Build history of the part. All positions in model axes, mm. A direction names the side the tool comes from. Round coordinates to 2 decimals unless told otherwise and drop trailing zeros. Write each loop counter-clockwise with the first axis right and the second up, starting at its lowest first coordinate (ties: lowest second). Pieces come first, ordered by that corner, then holes. Notation, with made-up numbers: M 49,60.25 L 81,60.25 A19 ccw 81,70.25 Z; hole C -30,70.25 d3. An arc over 180 degrees is marked long. Use a Markdown table: item, result.
from build123d import *

# Parameters (mm, degrees)
F0_W      = 1.5
F0_H      = 2
F0_H_2    = 12
F0_W_2    = 25
F0_H_3    = 16.5
F1_DEPTH  = 2
F2_DEPTH  = 12
F3_DEPTH  = 4
F4_DEPTH  = 7.97
F5_DEPTH  = 6
F6_SIZE2  = 5
F6_SIZE   = 3
F7_R      = 1
F8_DEPTH  = 15
F9_DEPTH  = 19
F10_DEPTH = 12.5


with BuildPart() as f1:
    # F0 (on Top) → F1 (new body)
    with BuildSketch(Plane.XY):
        Polygon((-5.2, 36.80300952), (-14, 24.80300952), (-12.5, 24.80300952), (-3.7, 36.80300952), align=None)
        Polygon((14, 24.80300952), (5.2, 36.80300952), (3.7, 36.80300952), (12.5, 24.80300952), align=None)
        Polygon((-12.5, 2.80300952), (-14, 2.80300952), (-14, -15.19699048), (14, -15.19699048), (14, 2.80300952), (12.5, 2.80300952), (12.5, -13.69699048), (-12.5, -13.69699048), align=None)
        with Locations((-13.25, 5.80300952)):
            Rectangle(F0_W, F0_H)
        with Locations((-13.25, 3.80300952)):
            Rectangle(F0_W, F0_H)
        with Locations((13.25, 5.80300952)):
            Rectangle(F0_W, F0_H)
        with Locations((13.25, 3.80300952)):
            Rectangle(F0_W, F0_H)
        with BuildLine():
            Line((-3, 39.80300952), (-5.2, 36.80300952))
            Line((-5.2, 36.80300952), (-3.7, 36.80300952))
            Line((-3.7, 36.80300952), (-1.5, 36.80300952))
            Line((-1.5, 36.80300952), (0, 36.80300952))
            Line((0, 36.80300952), (0, 38.30300952))
            ThreePointArc((0, 38.30300952), (-1.0606601718, 38.7423493483), (-1.5, 39.80300952))
            Line((-1.5, 39.80300952), (-3, 39.80300952))
        make_face()
        with BuildLine():
            Line((5.2, 36.80300952), (3, 39.80300952))
            Line((3, 39.80300952), (1.5, 39.80300952))
            ThreePointArc((1.5, 39.80300952), (1.0606601718, 38.7423493483), (0, 38.30300952))
            Line((0, 38.30300952), (0, 36.80300952))
            Line((0, 36.80300952), (1.5, 36.80300952))
            Line((1.5, 36.80300952), (3.7, 36.80300952))
            Line((3.7, 36.80300952), (5.2, 36.80300952))
        make_face()
        Polygon((-12.5, 24.80300952), (-14, 24.80300952), (-14, 6.80300952), (-12.5, 6.80300952), (-12.5, 23.30300952), (12.5, 23.30300952), (12.5, 6.80300952), (14, 6.80300952), (14, 24.80300952), (12.5, 24.80300952), (1.5, 24.80300952), (0, 24.80300952), (-1.5, 24.80300952), align=None)
        with Locations((0.75, 30.80300952)):
            Rectangle(F0_W, F0_H_2)
        with Locations((-0.75, 30.80300952)):
            Rectangle(F0_W, F0_H_2)
        with BuildLine():
            ThreePointArc((0, 38.30300952), (1.0606601718, 38.7423493483), (1.5, 39.80300952))
            Line((1.5, 39.80300952), (0, 39.80300952))
            Line((0, 39.80300952), (0, 38.30300952))
        make_face()
        with BuildLine():
            Line((0, 39.80300952), (-1.5, 39.80300952))
            ThreePointArc((-1.5, 39.80300952), (-1.0606601718, 38.7423493483), (0, 38.30300952))
            Line((0, 38.30300952), (0, 39.80300952))
        make_face()
        with Locations((0, 15.05300952)):
            Rectangle(F0_W_2, F0_H_3)
        with Locations((0, -5.44699048)):
            Rectangle(F0_W_2, F0_H_3)
        with Locations((0, 3.80300952)):
            Rectangle(F0_W_2, F0_H)
        with Locations((0, 5.80300952)):
            Rectangle(F0_W_2, F0_H)
        with BuildLine():
            ThreePointArc((3, 39.80300952), (0, 42.80300952), (-3, 39.80300952))
            Line((-3, 39.80300952), (-1.5, 39.80300952))
            ThreePointArc((-1.5, 39.80300952), (0, 41.30300952), (1.5, 39.80300952))
            Line((1.5, 39.80300952), (3, 39.80300952))
        make_face()
        with BuildLine():
            ThreePointArc((1.5, 39.80300952), (0, 41.30300952), (-1.5, 39.80300952))
            Line((-1.5, 39.80300952), (0, 39.80300952))
            Line((0, 39.80300952), (1.5, 39.80300952))
        make_face()
    extrude(amount=F1_DEPTH)

    # F0 (on Top) → F2 (join)
    with BuildSketch(Plane.XY):
        Polygon((-12.5, 2.80300952), (-14, 2.80300952), (-14, -15.19699048), (14, -15.19699048), (14, 2.80300952), (12.5, 2.80300952), (12.5, -13.69699048), (-12.5, -13.69699048), align=None)
        Polygon((-12.5, 24.80300952), (-14, 24.80300952), (-14, 6.80300952), (-12.5, 6.80300952), (-12.5, 23.30300952), (12.5, 23.30300952), (12.5, 6.80300952), (14, 6.80300952), (14, 24.80300952), (12.5, 24.80300952), (1.5, 24.80300952), (0, 24.80300952), (-1.5, 24.80300952), align=None)
        with Locations((13.25, 5.80300952)):
            Rectangle(F0_W, F0_H)
        with Locations((13.25, 3.80300952)):
            Rectangle(F0_W, F0_H)
        with Locations((-13.25, 3.80300952)):
            Rectangle(F0_W, F0_H)
        with Locations((-13.25, 5.80300952)):
            Rectangle(F0_W, F0_H)
    extrude(amount=F2_DEPTH)

    # F0 (on Top) → F3 (join)
    with BuildSketch(Plane.XY):
        with Locations((13.25, 5.80300952)):
            Rectangle(F0_W, F0_H)
        with Locations((13.25, 3.80300952)):
            Rectangle(F0_W, F0_H)
        with Locations((-13.25, 3.80300952)):
            Rectangle(F0_W, F0_H)
        with Locations((-13.25, 5.80300952)):
            Rectangle(F0_W, F0_H)
    extrude(amount=-F3_DEPTH)

    # F0 (on Top) → F4 (join)
    with BuildSketch(Plane.XY):
        with BuildLine():
            ThreePointArc((3, 39.80300952), (0, 42.80300952), (-3, 39.80300952))
            Line((-3, 39.80300952), (-1.5, 39.80300952))
            ThreePointArc((-1.5, 39.80300952), (0, 41.30300952), (1.5, 39.80300952))
            Line((1.5, 39.80300952), (3, 39.80300952))
        make_face()
        with BuildLine():
            ThreePointArc((1.5, 39.80300952), (0, 41.30300952), (-1.5, 39.80300952))
            Line((-1.5, 39.80300952), (0, 39.80300952))
            Line((0, 39.80300952), (1.5, 39.80300952))
        make_face()
        with BuildLine():
            Line((5.2, 36.80300952), (3, 39.80300952))
            Line((3, 39.80300952), (1.5, 39.80300952))
            ThreePointArc((1.5, 39.80300952), (1.0606601718, 38.7423493483), (0, 38.30300952))
            Line((0, 38.30300952), (0, 36.80300952))
            Line((0, 36.80300952), (1.5, 36.80300952))
            Line((1.5, 36.80300952), (3.7, 36.80300952))
            Line((3.7, 36.80300952), (5.2, 36.80300952))
        make_face()
        with BuildLine():
            Line((-3, 39.80300952), (-5.2, 36.80300952))
            Line((-5.2, 36.80300952), (-3.7, 36.80300952))
            Line((-3.7, 36.80300952), (-1.5, 36.80300952))
            Line((-1.5, 36.80300952), (0, 36.80300952))
            Line((0, 36.80300952), (0, 38.30300952))
            ThreePointArc((0, 38.30300952), (-1.0606601718, 38.7423493483), (-1.5, 39.80300952))
            Line((-1.5, 39.80300952), (-3, 39.80300952))
        make_face()
        with BuildLine():
            Line((-3, 49.80300952), (-3, 39.80300952))
            ThreePointArc((-3, 39.80300952), (0, 42.80300952), (3, 39.80300952))
            Line((3, 39.80300952), (3, 49.80300952))
            Line((3, 49.80300952), (1.5, 49.80300952))
            ThreePointArc((1.5, 49.80300952), (0, 48.30300952), (-1.5, 49.80300952))
            Line((-1.5, 49.80300952), (-3, 49.80300952))
        make_face()
        with BuildLine():
            ThreePointArc((3, 49.80300952), (0, 52.80300952), (-3, 49.80300952))
            Line((-3, 49.80300952), (-1.5, 49.80300952))
            ThreePointArc((-1.5, 49.80300952), (0, 51.30300952), (1.5, 49.80300952))
            Line((1.5, 49.80300952), (3, 49.80300952))
        make_face()
        with BuildLine():
            Line((0, 39.80300952), (-1.5, 39.80300952))
            ThreePointArc((-1.5, 39.80300952), (-1.0606601718, 38.7423493483), (0, 38.30300952))
            Line((0, 38.30300952), (0, 39.80300952))
        make_face()
        with BuildLine():
            ThreePointArc((0, 38.30300952), (1.0606601718, 38.7423493483), (1.5, 39.80300952))
            Line((1.5, 39.80300952), (0, 39.80300952))
            Line((0, 39.80300952), (0, 38.30300952))
        make_face()
    extrude(amount=-F4_DEPTH)

    # F0 (on Top) → F5 (cut)
    with BuildSketch(Plane.XY):
        with BuildLine():
            Line((-3, 49.80300952), (-3, 39.80300952))
            ThreePointArc((-3, 39.80300952), (0, 42.80300952), (3, 39.80300952))
            Line((3, 39.80300952), (3, 49.80300952))
            Line((3, 49.80300952), (1.5, 49.80300952))
            ThreePointArc((1.5, 49.80300952), (0, 48.30300952), (-1.5, 49.80300952))
            Line((-1.5, 49.80300952), (-3, 49.80300952))
        make_face()
        with BuildLine():
            ThreePointArc((3, 49.80300952), (0, 52.80300952), (-3, 49.80300952))
            Line((-3, 49.80300952), (-1.5, 49.80300952))
            ThreePointArc((-1.5, 49.80300952), (0, 51.30300952), (1.5, 49.80300952))
            Line((1.5, 49.80300952), (3, 49.80300952))
        make_face()
    extrude(amount=-F5_DEPTH, mode=Mode.SUBTRACT)

    # F6
    f6_edges = [f1.edges().sort_by_distance(p)[0] for p in [
        (0, 36.80301, -7.97),
    ]]
    f6_side = f1.faces().sort_by_distance((0, 43.604594, -7.97))[0]
    chamfer(f6_edges, length=F6_SIZE, length2=F6_SIZE2, reference=f6_side)

    # F7 (on Right) → F8 (cut, symmetric)
    with BuildSketch(Plane.YZ):
        with Locations((4.80300952, -2)):
            Circle(F7_R)
    extrude(amount=F8_DEPTH, both=True, mode=Mode.SUBTRACT)

    # F7 (on Right) → F9 (join, symmetric)
    with BuildSketch(Plane.YZ):
        Polygon((-9.3749196136, 0), (-8.19699048, 0), (-6.9519731405, 2), (-8.1299022741, 2), align=None)
        Polygon((-8.1299022741, 2), (-6.9519731405, 2), (-2.5944124523, 9), (12.4597597892, 9), (16.615620691, 2), (17.7785794425, 2), (13.0290241263, 10), (-3.1498329163, 10), align=None)
    extrude(amount=F9_DEPTH, both=True)

    # F7 (on Right) → F10 (cut, symmetric)
    with BuildSketch(Plane.YZ):
        Polygon((-8.1299022741, 2), (-6.9519731405, 2), (-2.5944124523, 9), (12.4597597892, 9), (16.615620691, 2), (17.7785794425, 2), (13.0290241263, 10), (-3.1498329163, 10), align=None)
    extrude(amount=F10_DEPTH, both=True, mode=Mode.SUBTRACT)


solid = f1.part
Q1. Drill centre lines: L1, parallel to X at y = 10, z = 10.5; L2, parallel to Y at x = -6, z = 4.25; L3, parallel to Y at x = -8, z = 0.75. Where is each one in solid material? Low to high.
Response values:
| item | result |
|---|---|
| L1 | x = -14 to -12.5, 12.5 to 14 |
| L2 | y = -15.2 to -13.7, 23.3 to 24.8 |
| L3 | y = -15.2 to 24.8, 30.94 to 32.98 |
Q2. Drop flat-ended pins along their axis: P1, Ø5.5, axis at x = 17.5, y = 3, coming from the +Z side; P2, Ø3.5, axis at x = -2.5, z = 9, coming from the +Y side; P3, Ø1.5, axis at x = 6, z = -4, coming from the +Y side; P4, Ø1, axis at y = 47.5, z = -7.5, coming from the -X side. Give the stop position or say it passes through.
Response values:
| item | result |
|---|---|
| P1 | stops at z = 10 |
| P2 | stops at y = 24.8 |
| P3 | passes through |
| P4 | stops at x = -3 |
Q3. Cut at B-B on z = -2. Give the cut face in (x, y).
Response values:
| item | result |
|---|---|
| outline | M -14,2.8 L -12.5,2.8 L -12.5,3.8 L -14,3.8 Z; M -14,5.8 L -12.5,5.8 L -12.5,6.8 L -14,6.8 Z; M -5.2,36.8 L 5.2,36.8 L 3,39.8 A3 ccw -3,39.8 Z; M 12.5,2.8 L 14,2.8 L 14,3.8 L 12.5,3.8 Z; M 12.5,5.8 L 14,5.8 L 14,6.8 L 12.5,6.8 Z |
Q4. Cut at C-C on y = 8. Give the cut face in (x, z), and give its area (3 significant figures).
Response values:
| item | result |
|---|---|
| outline | M -19,9 L -14,9 L -14,0 L 14,0 L 14,9 L 19,9 L 19,10 L 14,10 L 14,12 L 12.5,12 L 12.5,2 L -12.5,2 L -12.5,12 L -14,12 L -14,10 L -19,10 Z |
| area | 96.0 mm2 |
Q5. Cut at D-D on x = -15.5. Give the cut face in (y, z).
Response values:
| item | result |
|---|---|
| outline | M -9.37,0 L -8.2,0 L -2.59,9 L 12.46,9 L 16.62,2 L 17.78,2 L 13.03,10 L -3.15,10 Z |
Q6. Cut at A-A on x = 0. Give the cut face in (y, z).
Response values:
| item | result |
|---|---|
| outline | M -15.2,0 L 36.8,0 L 36.8,-2.97 L 39.8,-7.97 L 48.3,-7.97 L 48.3,-6 L 42.8,-6 L 42.8,2 L 24.8,2 L 24.8,12 L 23.3,12 L 23.3,2 L -13.7,2 L -13.7,12 L -15.2,12 Z; M 51.3,-7.97 L 52.8,-7.97 L 52.8,-6 L 51.3,-6 Z |
Q7. Two-plate mould, pull along Y, no slides. Class faces 1 (the flat face through (-16, 5, 10)), 2 (the flat face through (-13, 2.803, -2)), 3 (the flat face through (0, 5, 2)): +Y half, -Y half, draft (parallel to the pull), parting line (faces both ways), or undercut.
Response values:
| item | result |
|---|---|
| face 1 | draft |
| face 2 | -Y half |
| face 3 | undercut |
Q8. Which spindle directions (+Z, -Z, +X, -X, +Y, -Y) get a long thin tool onto all of the face, cutting with end or side? Do faces 4 (the flat face through (-12.5, 5, 7)), 5 (the flat face through (17, 5, 9)), 6 (the flat face through (1.5, 31, 1)), 7 (the flat face through (-16, 5, 9)). Say none if no direction does.
Response values:
| item | result |
|---|---|
| face 4 | +Z |
| face 5 | -Z, +X |
| face 6 | +Z, -Z |
| face 7 | -Z, -X |
